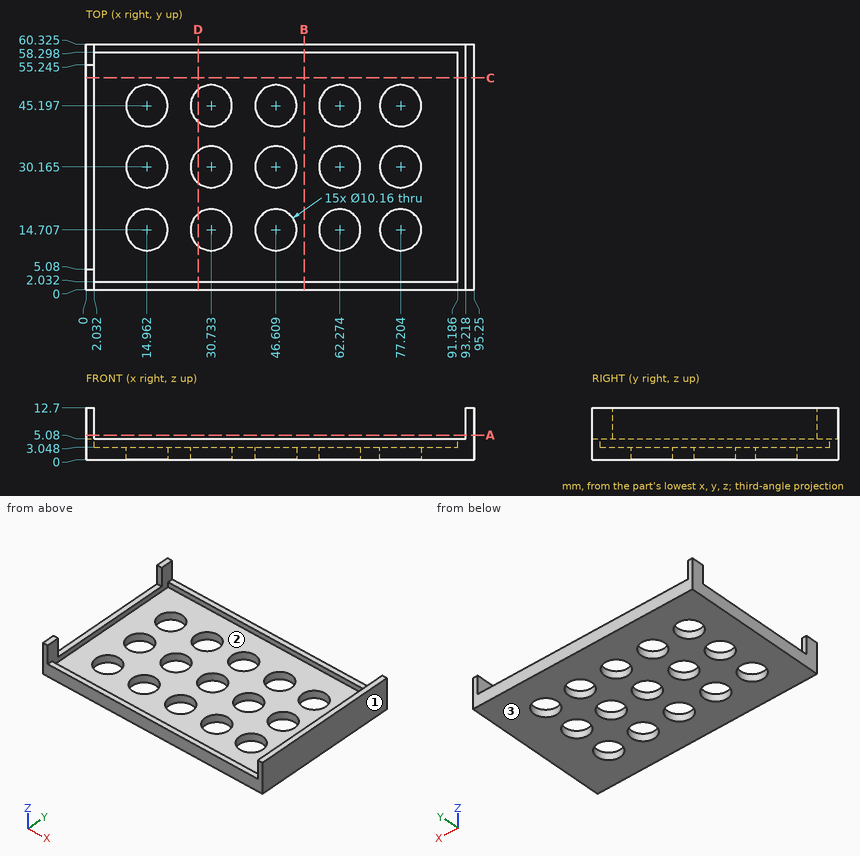
Drawing for the job (mm, zero at the part's lowest x, y, z). Round coordinates to 2 decimals unless told otherwise and drop trailing zeros. Write each loop counter-clockwise with the first axis right and the second up, starting at its lowest first coordinate (ties: lowest second). Pieces come first, ordered by that corner, then holes. Notation, with made-up numbers: M 14,-18 L 67,-18 A25 ccw 67,19 Z; hole C 52.5,20.5 d2. An arc over 180 degrees is marked long. Answer as a JSON object with one key per item and string values. Group by question number.
(1) Flat gauge pins, fed straight in: pin 1 (11.5 mm diameter, centred on x = 62.27, y = 30.16, fed in from +Z); pin 2 (2.5 mm diameter, centred on y = 29, z = 9, fed in from -X); pin 3 (2 mm diameter, centred on x = 1, y = 31, fed in from +Z). Where does each tip first touch, or does it go through?
(2) Cut at A-A (z = 6). Give the number of separate pieces and of enclosed holes in the cut face, and give its area (3 significant figures).
(3) Mould opens along X. For the marked faces 1, 2 and 3 say: pulls with the +X half, pulls with the -X half, needs draft (parallel to the pull), parting line crosses it, or undercut.
(4) Drill centre lines: L1, parallel to Y at x = 62, z = 2.75 (1 decimal); L2, parallel to Y at x = 84, z = 3.5 (1 decimal); L3, parallel to X at y = 56.5, z = 5.25. Where is each one in solid material? Low to high.
(5) Cut at D-D (x = 27.5). Give the cut face in (y, z) (1 decimal).
(6) Cut at C-C (y = 52). Give the cut face in (x, z), and give its area (3 significant figures).
(7) Cut at B-B (x = 53.5). Give the cut face in (y, z) (1 decimal), and give its area (3 significant figures).
Responses:
{
 "1": {"pin 1": "stops at z = 3.05", "pin 2": "stops at x = 93.22", "pin 3": "stops at z = 5.08"},
 "2": {"separate pieces": "3", "enclosed holes": "0", "area": "143 mm2"},
 "3": {"face 1": "pulls with the +X half", "face 2": "undercut", "face 3": "needs draft"},
 "4": {"L1": "y = 0 to 9.6, 19.8 to 25.1, 35.2 to 40.1, 50.3 to 60.3", "L2": "y = 0 to 2, 58.3 to 60.3", "L3": "x = 0 to 2.03, 93.22 to 95.25"},
 "5": {"outline": "M 0,0 L 10.8,0 L 10.8,3 L 2,3 L 2,5.1 L 0,5.1 Z; M 18.6,0 L 26.2,0 L 26.2,3 L 18.6,3 Z; M 34.1,0 L 41.3,0 L 41.3,3 L 34.1,3 Z; M 49.1,0 L 60.3,0 L 60.3,5.1 L 58.3,5.1 L 58.3,3 L 49.1,3 Z"},
 "6": {"outline": "M 0,0 L 95.25,0 L 95.25,12.7 L 93.22,12.7 L 93.22,5.08 L 91.19,5.08 L 91.19,3.05 L 2.03,3.05 L 2.03,5.08 L 0,5.08 Z", "area": "318 mm2"},
 "7": {"outline": "M 0,0 L 60.3,0 L 60.3,5.1 L 58.3,5.1 L 58.3,3 L 2,3 L 2,5.1 L 0,5.1 Z", "area": "192 mm2"}
}
